Design review of the part built by this model. Coordinates are the model's own, in mm. Round coordinates to 2 decimals unless told otherwise and drop trailing zeros. Order: outer loops, then holes, each group sorted by start corner. A loop starts at its lowest first (then second) coordinate and runs counter-clockwise, first axis right, second up. Notation, with made-up numbers: (21, 39) - (53, 39) arc R21 cw to (53, 63) - close; hole circle Ø8 at (-9.75, -12). An arc over 180 degrees is marked (long way). Use CSV: the item, a comma, the result in double quotes.
from build123d import *

# Parameters (mm, degrees)
CUT_EXTRUDE1_REACH = 1549.869
SKETCH3_R          = 11
SKETCH4_R          = 32
CUT_EXTRUDE2_DEPTH = 500


with BuildPart() as part:
    # Sketch1 → Revolve1 (revolve)
    with BuildSketch(Plane.XY):
        with BuildLine():
            Line((0, 759), (0, 775))
            ThreePointArc((0, 775), (548.00775542, 548.00775542), (775, 0))
            Line((775, 0), (759, 0))
            ThreePointArc((759, 0), (536.694046921, 536.694046921), (0, 759))
        make_face()
    revolve(axis=Axis((0, 0, 0), (0, 1, 0)))

    # Sketch2 → Revolve2 (revolve)
    with BuildSketch(Plane.XY):
        Polygon((105, 1093), (105, 1061), (52.624014674, 1061), (38, 1010), (38, 774.067826486), (32, 774.067826486), (32, 1093), align=None)
    revolve(axis=Axis((0, 775, 0), (0, 1, 0)))

    # Sketch3 → Cut-Extrude1 (cut, up to next)
    with BuildSketch(Plane(origin=(0, 1093, 0), x_dir=(1, 0, 0), z_dir=(0, 1, 0)), mode=Mode.PRIVATE) as cut_extrude1_sk1:
        with Locations(Location((-80, 0, 0), (0, 0, 180))):
            Circle(SKETCH3_R)
    cut_extrude1_tool1 = extrude(cut_extrude1_sk1.sketch, amount=-CUT_EXTRUDE1_REACH, mode=Mode.PRIVATE) & part.part
    # Sketch3 → Cut-Extrude1 (cut, up to next)
    with BuildSketch(Plane(origin=(0, 1093, 0), x_dir=(1, 0, 0), z_dir=(0, 1, 0)), mode=Mode.PRIVATE) as cut_extrude1_sk2:
        with Locations(Location((80, 0, 0), (0, 0, 180))):
            Circle(SKETCH3_R)
    cut_extrude1_tool2 = extrude(cut_extrude1_sk2.sketch, amount=-CUT_EXTRUDE1_REACH, mode=Mode.PRIVATE) & part.part
    add(cut_extrude1_tool1.solids().sort_by_distance((-80, 1093, 0))[0], mode=Mode.SUBTRACT)
    add(cut_extrude1_tool2.solids().sort_by_distance((80, 1093, 0))[0], mode=Mode.SUBTRACT)

    # Sketch4 → Cut-Extrude2 (cut)
    with BuildSketch(Plane(origin=(0, 1093, 0), x_dir=(1, 0, 0), z_dir=(0, 1, 0))):
        Circle(SKETCH4_R)
    extrude(amount=-CUT_EXTRUDE2_DEPTH, mode=Mode.SUBTRACT)


solid = part.part
1) We need section A-A (x = 0). Give the boundary of the cut face in (y, z), then the cut area to 3 significant figures.
Data:
outline,"(0, -775) arc R775 ccw to (774.07, -38) - (1010, -38) - (1061, -52.62) - (1061, -105) - (1093, -105) - (1093, -32) - (758.33, -32) arc R759 cw to (0, -759) - close; (0, 759) arc R759 cw to (758.33, 32) - (1093, 32) - (1093, 105) - (1061, 105) - (1061, 52.62) - (1010, 38) - (774.07, 38) arc R775 ccw to (0, 775) - close"
area,"46,400 mm2"
2) The part is to be moulded in two halves that separate along Y. For faces 1 (the face through (-33.3, 1023.81, 25.53)), 2 (the face through (100.15, 1076.78, -31.54)), 3 (the face through (-22, 1093, -25)), 4 (the face through (570, 0, 513)), say which applies: +Y half, -Y half, draft (parallel to the pull), parting line (faces both ways), or undercut.
Data:
face 1,"undercut"
face 2,"draft"
face 3,"+Y half"
face 4,"-Y half"
3) We need section B-B (y = 813). Give the boundary of the cut face in (x, z), then the cut area to 3 significant figures.
Data:
outline,"circle Ø76 at (0, 0); hole circle Ø64 at (0, 0)"
area,"1,320 mm2"
4) We need section C-C (z = 417). Give the boundary of the cut face in (x, y), then the cut area to 3 significant figures.
Data:
outline,"(-653.25, 0) - (-634.19, 0) arc R634.19 cw to (634.19, 0) - (653.25, 0) arc R653.25 ccw to start"
area,"38,600 mm2"
5) To check wall thickness, follow L1, parallel to Z at x = 0, y = 953; L2, parallel to Z at x = -579, y = 217.5; L3, parallel to X at y = 180, z = -33.5. State the ranges of each line that lie inside material, in increasing order. Write a range as from..to.
Data:
L1,"z = -38..-32, 32..38"
L2,"z = -466.99..-439.92, 439.92..466.99"
L3,"x = -753.06..-736.59, 736.59..753.06"
6) Insertion check: pin 1 Ø3 at (x, z) = (-278.5, -506) entering from -Y; pin 2 Ø12 at (x, y) = (107, 445) entering from +Z; pin 3 Ø1 at (x, y) = (-286.5, 628) entering from -Z. Each pin has a flat end and moves straight along its axis. Give the tip position at first contact, or say it passes through.
Data:
pin 1,"stops at y = 490.66"
pin 2,"stops at z = 629.77"
pin 3,"stops at z = -353.34"
